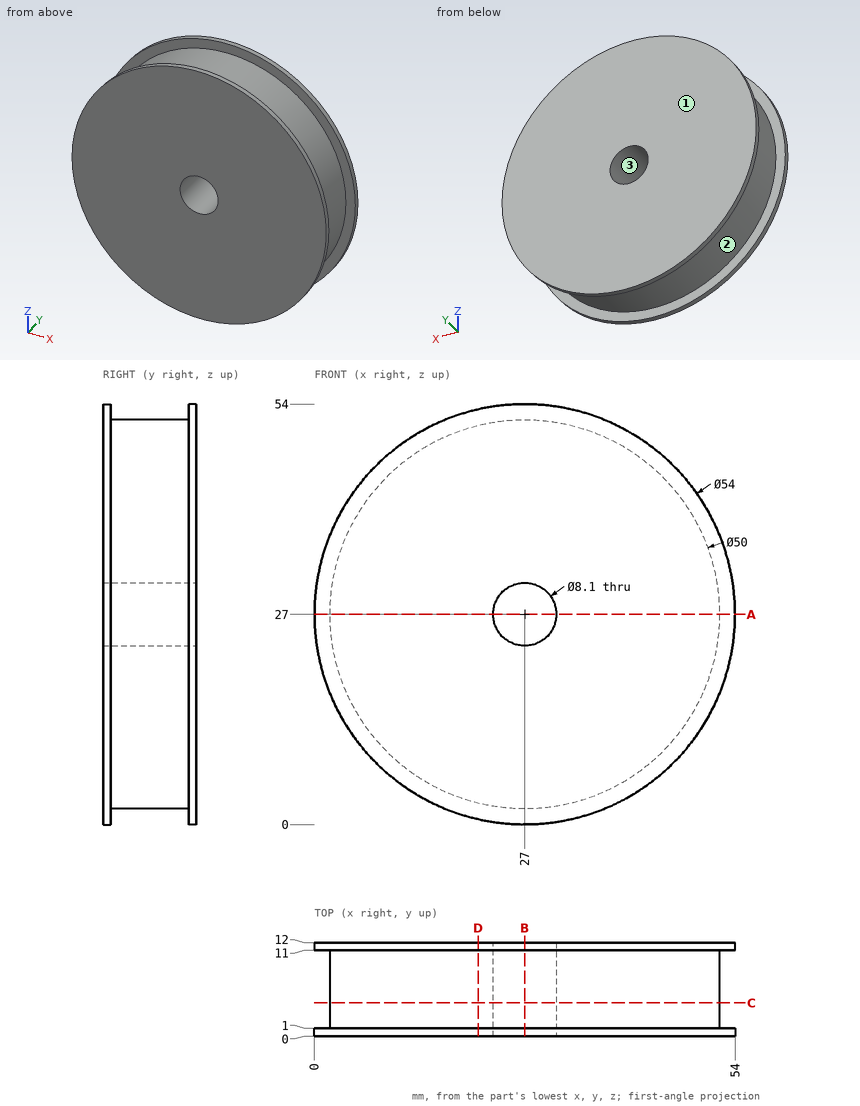
Could you check a few things on this drawing? It's one solid part, dimensions in mm from its lowest x, y, z. Give positions to 0.01 mm unless a question says otherwise; leave off trailing zeros. Write each loop counter-clockwise with the first axis right and the second up, starting at its lowest first coordinate (ties: lowest second). Pieces come first, ordered by that corner, then holes. Notation, with made-up numbers: (41.5, 37) -> (99.5, 37) arc R22 ccw to (99.5, 75) -> close; hole circle Ø8 at (-13, -32.75). An arc over 180 degrees is marked (long way). Answer as a JSON object with one key per item and string values.
Q1. Suppose I cut it at A-A on z = 27. Write out the boundary of the cut face in (x, y).
Taken from the geometry:
{"outline": "(0, 0) -> (22.95, 0) -> (22.95, 12) -> (0, 12) -> (0, 11) -> (2, 11) -> (2, 1) -> (0, 1) -> close; (31.05, 0) -> (54, 0) -> (54, 1) -> (52, 1) -> (52, 11) -> (54, 11) -> (54, 12) -> (31.05, 12) -> close"}
Q2. Suppose I cut it at C-C on y = 4.25. Write out the boundary of the cut face in (x, z).
Taken from the geometry:
{"outline": "circle Ø50 at (27, 27); hole circle Ø8.1 at (27, 27)"}
Q3. We'd pull the mould along Y, two halves only. Please class the marked faces 1, 2 and 3: released by +Y, released by -Y, zero draft, split by the parting line, or undercut.
Taken from the geometry:
{"face 1": "released by +Y", "face 2": "undercut", "face 3": "zero draft"}
Q4. Suppose I cut it at B-B on x = 27. Write out the boundary of the cut face in (y, z).
Taken from the geometry:
{"outline": "(0, 0) -> (1, 0) -> (1, 2) -> (11, 2) -> (11, 0) -> (12, 0) -> (12, 22.95) -> (0, 22.95) -> close; (0, 31.05) -> (12, 31.05) -> (12, 54) -> (11, 54) -> (11, 52) -> (1, 52) -> (1, 54) -> (0, 54) -> close"}
Q5. Suppose I cut it at D-D on x = 21. Write out the boundary of the cut face in (y, z), then the cut area to 3 significant figures.
Taken from the geometry:
{"outline": "(0, 0.68) -> (1, 0.68) -> (1, 2.73) -> (11, 2.73) -> (11, 0.68) -> (12, 0.68) -> (12, 53.32) -> (11, 53.32) -> (11, 51.27) -> (1, 51.27) -> (1, 53.32) -> (0, 53.32) -> close", "area": "591 mm²"}
Q6. Will these pins go through, and if not, where does the flat tip stop? pin 1 Ø7.5 at (x, z) = (27, 27) entering from +Y; pin 2 Ø4 at (y, z) = (9.5, 47.5) entering from -X; pin 3 Ø6 at (y, z) = (10, 31) entering from +X; pin 4 Ø3 at (y, z) = (7.5, 18.5) entering from -X.
Taken from the geometry:
{"pin 1": "passes through", "pin 2": "stops at x = 7.99", "pin 3": "stops at x = 53.97", "pin 4": "stops at x = 3"}
Q7. Please list where these lines run through material, in increasing order: L1, parallel to Y at x = 20.5, z = 51.5; L2, parallel to Z at x = 27, y = 5; L3, parallel to X at y = 11.5, z = 27.5.
Taken from the geometry:
{"L1": "y = 0 to 1, 11 to 12", "L2": "z = 2 to 22.95, 31.05 to 52", "L3": "x = 0 to 22.98, 31.02 to 54"}
